Part print with two shaded views. Sizes in mm from the minimum x, y, z corner. Give positions to 0.01 mm unless a question says otherwise; leave off trailing zeros. Loops run counter-clockwise (first coordinate to the right, second up) from the corner with the lowest first, then second, coordinate; pieces in that order, holes last. Notation, with made-up numbers: M 22.25,30 L 66.25,30 A26 cw 66.25,69 Z; hole C 30.5,31 d7. An arc over 180 degrees is marked long. Answer as a JSON object with one key per item and string values. Group by question number.
1. Mould opens along X. For the marked faces 1, 2 and 3 say: released by +X, released by -X, zero draft, split by the parting line, or undercut.
2. Drop flat-ended pins along their axis: pin 1 Ø12 at (x, y) = (38, 60.5) entering from +Z; pin 2 Ø5 at (x, z) = (45.5, 86.5) entering from -Y; pin 3 Ø1.5 at (x, z) = (11.5, 33.5) entering from -Y; pin 4 Ø7.5 at (y, z) = (50.8, 50.8) entering from -X. Give the stop position or say it passes through.
3. Slice it at A-A (z = 50.8). List the corners of the cut face in (x, y) (3 decimals), then the cut area to 3 significant figures.
4. Drill centre lines: line 1 along Z through (x, y) = (13, 50.8); line 2 along X through (y, z) = (24.5, 14.5). Where is each one in solid material? Low to high. Write a range as [from, to].
5. Slice it at C-C (x = 17.5). List the corners of the cut face in (y, z).
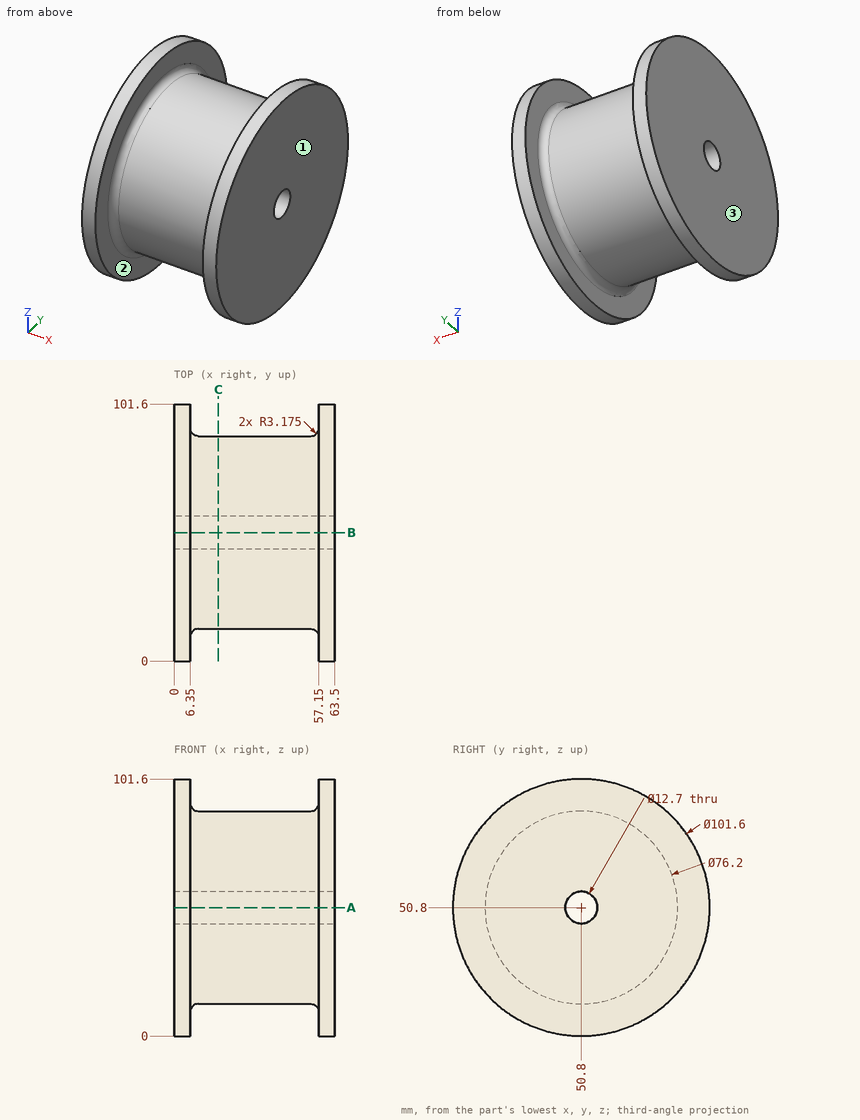
Established:
{
 "1": {"face 1": "released by +X", "face 2": "undercut", "face 3": "released by -X"},
 "2": {"pin 1": "stops at z = 88.72", "pin 2": "stops at y = 32.11", "pin 3": "stops at y = 16.48", "pin 4": "passes through"},
 "3": {"outline": "M 0,0 L 6.35,0 L 6.35,9.525 A3.175 cw 9.525,12.7 L 53.975,12.7 A3.175 cw 57.15,9.525 L 57.15,0 L 63.5,0 L 63.5,44.45 L 0,44.45 Z; M 0,57.15 L 63.5,57.15 L 63.5,101.6 L 57.15,101.6 L 57.15,92.075 A3.175 cw 53.975,88.9 L 9.525,88.9 A3.175 cw 6.35,92.075 L 6.35,101.6 L 0,101.6 Z", "area": "4,360 mm^2"},
 "4": {"line 1": "z = [12.7, 44.45], [57.15, 88.9]", "line 2": "x = [0, 6.35], [57.15, 63.5]"},
 "5": {"outline": "C 50.8,50.8 d76.2; hole C 50.8,50.8 d12.7"}
}
